The listing builds one solid part. Answer for the finished solid, in the listing's coordinates (mm). Face numbers are marked on the shaded views. Round coordinates to 2 decimals unless told otherwise and drop trailing zeros. Write each loop counter-clockwise with the first axis right and the second up, starting at its lowest first coordinate (ties: lowest second). Pieces come first, ordered by that corner, then holes.
Item 1: Find section A-A on z = 35. Give the vertices of the cut face in (x, y).
Item 2: Find section B-B on x = 0. Give the vertices of the cut face in (y, z), then the cut area to 3 significant figures.
Item 3: Find the intervals of material crossed by probe 1 along X at (y, z) = (-1.5, 8.5) (3 decimals); probe 2 along Z at (x, y) = (18.5, -59); probe 3 along X at (y, z) = (-2, 8), in increasing order.
Item 4: Find section D-D on y = -36.5. Give the vertices of the cut face in (x, z), then the cut area to 3 significant figures.
Item 5: Each of these flat-tipped pins is pushed along its axis until it touches: pin 1 (1.2 mm diameter, centred on y = -2.5, z = 9, fed in from +X); pin 2 (1.2 mm diameter, centred on x = -46.5, y = -2, fed in from +Z); pin 3 (12 mm diameter, centred on y = -9.5, z = 11, fed in from +X). Where does it stop, or does it pass through?
Item 6: For a pull along X with two mould halves and no side action, classify the marked faces 1, 2 and 3 as +X half, -X half, draft (parallel to the pull), parting line (faces both ways), or undercut.
Item 7: Find section C-C on x = -47.5. Give the vertices of the cut face in (y, z), then the cut area to 3 significant figures.
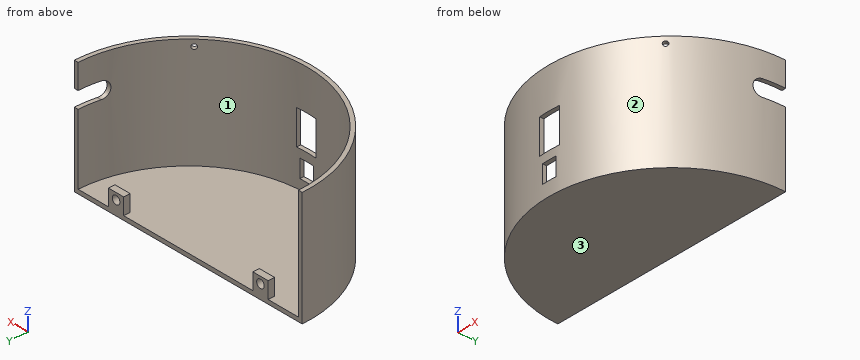
```python
from build123d import *

# Parameters (mm, degrees)
SZKIC1_R                         = 75
DODANIE_WYCI_GNI_CIE1_DEPTH      = 70
SKORUPA1_T                       = -2.5
SZKIC3_W                         = 13
SZKIC3_H                         = 21
WYTNIJ_WYCI_GNI_CIE1_DEPTH       = 60
SZKIC4_W                         = 9
SZKIC4_H                         = 11
WYTNIJ_WYCI_GNI_CIE2_DEPTH       = 60
DODANIE_WYCI_GNI_CIE2_REACH      = 192.066
DODANIE_WYCI_GNI_CIE2_END_RADIUS = 75
SZKIC7_W                         = 60
SZKIC7_H                         = 35
SZKIC8_W                         = 45.5
SZKIC8_H                         = 26.5
WYTNIJ_WYCI_GNI_CIE4_DEPTH       = 30
ZAOKR_GLENIE1_R                  = 5
WYTNIJ_WYCI_GNI_CIE5_DEPTH       = 14
SZKIC10_R                        = 1.5
WYTNIJ_WYCI_GNI_CIE6_DEPTH       = 10
SZYK_KO_OWY1_COUNT               = 4
PRZECI_CIE2_OUTLINE_W            = 152
PRZECI_CIE2_OUTLINE_H            = 70
PRZECI_CIE2_OUTLINE_W_2          = 45.5
PRZECI_CIE2_OUTLINE_H_2          = 26.5
PRZECI_CIE2_DEPTH                = 85
SZKIC11_W                        = 10
SZKIC11_H                        = 10
SZKIC11_R                        = 2.5
DODANIE_WYCI_GNI_CIE3_DEPTH      = 4


# Read off the part's stored shape, not the designer's step: Przecięcie2
with BuildPart() as part:
    # Szkic1 → Dodanie-wyciągnięcie1 (new body)
    with BuildSketch(Plane.XY):
        Circle(SZKIC1_R)
    extrude(amount=DODANIE_WYCI_GNI_CIE1_DEPTH)

    # Skorupa1
    skorupa1_openings = [part.faces().sort_by_distance(p)[0] for p in [
        (0, 0, 70),
    ]]
    offset(amount=SKORUPA1_T, openings=skorupa1_openings, kind=Kind.INTERSECTION)

    # Szkic3 → Wytnij-wyciągnięcie1 (cut)
    with BuildSketch(Plane(origin=(0, -75, 0), x_dir=(-1, 0, 0), z_dir=(0, -1, 0))):
        with Locations((0, -35)):
            Rectangle(SZKIC3_W, SZKIC3_H)
    extrude(amount=-WYTNIJ_WYCI_GNI_CIE1_DEPTH, mode=Mode.SUBTRACT)

    # Szkic4 → Wytnij-wyciągnięcie2 (cut)
    with BuildSketch(Plane(origin=(0, -75, 0), x_dir=(-1, 0, 0), z_dir=(0, -1, 0))):
        with Locations((0, -14)):
            Rectangle(SZKIC4_W, SZKIC4_H)
    extrude(amount=-WYTNIJ_WYCI_GNI_CIE2_DEPTH, mode=Mode.SUBTRACT)

    # Dodanie-wyciągnięcie2: up to this cylinder (the profile starts outside it)
    dodanie_wyci_gni_cie2_end = Plane(origin=(0, 0, 35.532003), z_dir=(0, 0, -1)) * Cylinder(DODANIE_WYCI_GNI_CIE2_END_RADIUS, 535.132, mode=Mode.PRIVATE)
    # Szkic7 → Dodanie-wyciągnięcie2 (add, up to the surface)
    with BuildSketch(Plane(origin=(0, 85, 0), x_dir=(-1, 0, 0), z_dir=(0, -1, 0)), mode=Mode.PRIVATE) as dodanie_wyci_gni_cie2_sk1:
        with Locations((0, -35.532003496)):
            Rectangle(SZKIC7_W, SZKIC7_H)
    dodanie_wyci_gni_cie2_tool1 = extrude(dodanie_wyci_gni_cie2_sk1.sketch, amount=DODANIE_WYCI_GNI_CIE2_REACH, mode=Mode.PRIVATE) - dodanie_wyci_gni_cie2_end
    add(dodanie_wyci_gni_cie2_tool1.solids().sort_by_distance((0, 85, 35.532003))[0])

    # Szkic8 → Wytnij-wyciągnięcie4 (cut)
    with BuildSketch(Plane(origin=(0, 85, 0), x_dir=(1, 0, 0), z_dir=(0, 1, 0))):
        with Locations((0, -35.532003496)):
            Rectangle(SZKIC8_W, SZKIC8_H)
    extrude(amount=-WYTNIJ_WYCI_GNI_CIE4_DEPTH, mode=Mode.SUBTRACT)

    # Zaokrąglenie1
    zaokr_glenie1_edges = [part.edges().sort_by_distance(p)[0] for p in [
        (-30, 76.869317712, 18.032003496),
        (-30, 76.869317712, 53.032003496),
        (30, 76.869317712, 18.032003496),
        (30, 76.869317712, 53.032003496),
    ]]
    fillet(zaokr_glenie1_edges, radius=ZAOKR_GLENIE1_R)

    # Szkic9 → Wytnij-wyciągnięcie5 (cut)
    with BuildSketch(Plane(origin=(75, 0, 0), x_dir=(0, 0, -1), z_dir=(1, 0, 0))):
        with BuildLine():
            Line((-55, -12.979686846), (-55, 12.020313154))
            ThreePointArc((-55, 12.020313154), (-50, 17.020313154), (-45, 12.020313154))
            Line((-45, 12.020313154), (-45, -12.979686846))
            ThreePointArc((-45, -12.979686846), (-50, -17.979686846), (-55, -12.979686846))
        make_face()
    extrude(amount=-WYTNIJ_WYCI_GNI_CIE5_DEPTH, mode=Mode.SUBTRACT)

    # Szkic10 → Wytnij-wyciągnięcie6 (cut)
    with BuildSketch(Plane(origin=(53.033008589, 53.033008589, 0), x_dir=(0, 0, -1), z_dir=(0.7071067811865512, 0.7071067811865438, 0))):
        with Locations(Location((-66, 0, 0), (0, 0, 90))):
            Circle(SZKIC10_R)
    wytnij_wyci_gni_cie6 = extrude(amount=-WYTNIJ_WYCI_GNI_CIE6_DEPTH, mode=Mode.SUBTRACT)

    # Szyk kołowy1: Wytnij-wyciągnięcie6 ×4 about axis
    szyk_ko_owy1_axis = Axis((0, 0, 70), (0, 0, -1))
    for i in range(1, SZYK_KO_OWY1_COUNT):
        add(wytnij_wyci_gni_cie6.rotate(szyk_ko_owy1_axis, i * 360 / SZYK_KO_OWY1_COUNT), mode=Mode.SUBTRACT)

    # Przecięcie2 outline → Przecięcie2 (cut)
    with BuildSketch(Plane(origin=(0, 0, 0), x_dir=(1, 0, 0), z_dir=(0, 1, 0))):
        with Locations((0, -35)):
            Rectangle(PRZECI_CIE2_OUTLINE_W, PRZECI_CIE2_OUTLINE_H)
        with Locations((0, -35.532003496)):
            Rectangle(PRZECI_CIE2_OUTLINE_W_2, PRZECI_CIE2_OUTLINE_H_2, mode=Mode.SUBTRACT)
    extrude(amount=PRZECI_CIE2_DEPTH, mode=Mode.SUBTRACT)

    # Szkic11 → Dodanie-wyciągnięcie3 (add)
    # profile 1 of 2: a face of its own
    with BuildSketch(Plane(origin=(0, 0, 0), x_dir=(1, 0, 0), z_dir=(0, 1, 0))):
        with Locations((47.5, -7.5)):
            Rectangle(SZKIC11_W, SZKIC11_H)
        with Locations(Location((47.5, -8.5, 0), (0, 0, 270))):
            Circle(SZKIC11_R, mode=Mode.SUBTRACT)
    # profile 2 of 2: a face of its own
    with BuildSketch(Plane(origin=(0, 0, 0), x_dir=(1, 0, 0), z_dir=(0, 1, 0))):
        with Locations((-47.5, -7.5)):
            Rectangle(SZKIC11_W, SZKIC11_H)
        with Locations(Location((-47.5, -8.5, 0), (0, 0, 270))):
            Circle(SZKIC11_R, mode=Mode.SUBTRACT)
    extrude(amount=-DODANIE_WYCI_GNI_CIE3_DEPTH)


solid = part.part
```
Check values:
1. outline: (-75, 0) arc R75 ccw to (-6.5, -74.72) - (-6.5, -72.21) arc R72.5 cw to (-72.5, 0) - close; (6.5, -74.72) arc R75 ccw to (75, 0) - (72.5, 0) arc R72.5 cw to (6.5, -72.21) - close
2. outline: (-75, 0) - (0, 0) - (0, 2.5) - (-72.5, 2.5) - (-72.5, 8.5) - (-75, 8.5) - close; (-75, 19.5) - (-72.5, 19.5) - (-72.5, 24.5) - (-75, 24.5) - close; (-75, 45.5) - (-72.5, 45.5) - (-72.5, 70) - (-75, 70) - close
2. area: 276 mm2
3. probe 1: x = -74.985 to -72.484, -52.5 to -50, -45 to -42.5, 42.5 to 45, 50 to 52.5, 72.484 to 74.985
3. probe 2: z = 0 to 2.5
3. probe 3: x = -74.97 to -72.47, -52.5 to -49.95, -45.05 to -42.5, 42.5 to 45.05, 49.95 to 52.5, 72.47 to 74.97
4. outline: (-65.52, 0) - (65.52, 0) - (65.52, 70) - (62.64, 70) - (62.64, 2.5) - (-62.64, 2.5) - (-62.64, 70) - (-65.52, 70) - close
4. area: 716 mm2
5. pin 1: stops at x = 74.98
5. pin 2: stops at z = 12.5
5. pin 3: stops at x = 74.92
6. face 1: undercut
6. face 2: parting line
6. face 3: draft
7. outline: (-58.04, 0) - (0, 0) - (0, 6) - (-4, 6) - (-4, 2.5) - (-54.77, 2.5) - (-54.77, 70) - (-58.04, 70) - close; (-4, 11) - (0, 11) - (0, 12.5) - (-4, 12.5) - close
7. area: 386 mm2
